Autodesk Inventor part; units mm, degrees
ref_plane "YZ Plane" through (0, 0, 0) normal (1, 0, 0) x (0, 1, 0)
ref_plane "XZ Plane" through (0, 0, 0) normal (0, 1, 0) x (-1, 0, 0)
ref_plane "XY Plane" through (0, 0, 0) normal (0, 0, 1) x (1, 0, 0)
sketch "Motor_Lego_Axle_Connector" plane through (0, 0, 0) normal (0, 0, 1) x (1, 0, 0)
  circle A0 centre (0, 0) radius 4.5
  circle A1 centre (0, 0) radius 2.7
  line L0 (-1.8, 2.0125) -> (-1.8, -2.0125)
  line L1 (0, 4.5) -> (0, -4.5) construction
  line L2 (1.8, 2.0125) -> (1.8, -2.0125)
  line L3 (0.9, 2.4) -> (-0.9, 2.4)
  line L4 (0.9, 2.4) -> (0.9, 1.4)
  line L5 (1.4, 1.4) -> (0.9, 1.4) construction
  line L6 (1.4, 1.4) -> (1.4, 0.9) construction
  arc A2 (0.9, 1.4) -> (1.4, 0.9) centre (1.4, 1.4) ccw
  line L7 (1.4, 0.9) -> (2.4, 0.9)
  line L8 (-0.9, 1.4) -> (-0.9, 2.4)
  arc A3 (-1.4, 0.9) -> (-0.9, 1.4) centre (-1.4, 1.4) ccw
  line L9 (-2.4, 0.9) -> (-1.4, 0.9)
  line L10 (-2.4, 0.9) -> (-2.4, -0.9)
  line L11 (-1.4, -0.9) -> (-2.4, -0.9)
  arc A4 (-0.9, -1.4) -> (-1.4, -0.9) centre (-1.4, -1.4) ccw
  line L12 (-0.9, -2.4) -> (-0.9, -1.4)
  line L13 (-0.9, -2.4) -> (0.9, -2.4)
  line L14 (0.9, -1.4) -> (0.9, -2.4)
  arc A5 (1.4, -0.9) -> (0.9, -1.4) centre (1.4, -1.4) ccw
  line L15 (2.4, -0.9) -> (1.4, -0.9)
  line L16 (2.4, -0.9) -> (2.4, 0.9)
  point P0 (1.8, -2.0125)
  point P1 (0, 2.4)
  point P2 (-2.4, 0)
  point P3 (0, -2.4)
  point P4 (2.4, 0)
  dimension "d0" = 9
  dimension "d1" = 5.4
  dimension "d2" = 9
  dimension "d3" = 1.8
  dimension "d12" = 1.8
  dimension "d13" = 2.4
  dimension "d14" = 1
  dimension "d16" = 0.5
  dimension "d17" = 1
  dimension "d20" = 360
extrude "Motor_Side_Outer_Ring_Extrusion" add sketch "Motor_Lego_Axle_Connector" along normal blind 9
extrude "Motor_Connector_Extrusion" add sketch "Motor_Lego_Axle_Connector" along normal blind 7.9 separate body contours A1 L2 L15 L16 L7 | L0 L9 L10 L11 A1 | L7 L16 L15 L2 | L0 L11 L10 L9
extrude "Seperation_Extrusion" add sketch "Motor_Lego_Axle_Connector" against normal blind 3 contours A1 L2 L15 L16 L7 | L2 L7 A2 L4 L3 L8 A3 L9 L0 A1 | A1 L0 L11 A4 L12 L13 L14 A5 L15 L2 | L0 L9 L10 L11 A1 | L7 L16 L15 L2 | L2 L15 A5 L14 L13 L12 A4 L11 L0 L9 A3 L8 L3 L4 A2 L7 | L0 L11 L10 L9
extrude "Lego_Axle_Side_Outer_Ring_Extrusion" add sketch "Motor_Lego_Axle_Connector" against normal blind 11
extrude "Lego_Axle_Connector_Extrusion" add sketch "Motor_Lego_Axle_Connector" against normal blind 11 contours A1 L2 L15 L16 L7 | L2 L7 A2 L4 L3 L8 A3 L9 L0 A1 | A1 L0 L11 A4 L12 L13 L14 A5 L15 L2 | L0 L9 L10 L11 A1
equation "\"d2\" = d0"
properties part number "Motor_Lego_Axle_Connector"
Source: CAD feature listing. Evaluate the final solid. Frame: model axes, mm. A direction names the side the tool comes from. Coordinates: 2 decimals unless noted, no trailing zeros. Loops run counter-clockwise (first coordinate to the right, second up) from the corner with the lowest first, then second, coordinate; pieces in that order, holes last. Notation, with made-up numbers: (43, 72) -> (92, 72) arc R29 cw to (92, 98) -> close; hole circle Ø8 at (48.5, -5). An arc over 180 degrees is marked (long way). One line per item, written item: value. Start each with the question number.
Q1. Section query C-C, the plane x = 0. Return the cut outline in (y, z), and give its area (3 significant figures).
Q2. Section query D-D, the plane z = -0.75. Return the cut outline in (x, y), and give its area (3 significant figures).
Q3. Line query: line 1 along Y through (x, z) = (0, 7); line 2 along X through (y, z) = (2.25, 6.75); line 3 along X through (y, z) = (-0.75, 5.75). Output: solid intervals per line, ascending.
Q4. Mould query, pull axis X, two halves, no side actions, for faces 4 (the face through (-0.59, 4.46, -0.86)), 5 (the face through (-0.9, 2, -7)), 6 (the face through (-1.1, -1.9, -11)). Classes: pulls with the +X half, pulls with the -X half, needs draft (parallel to the pull), parting line crosses it, or undercut.
Q5. Section query A-A, the plane z = -6.5. Return the cut outline in (x, y), and give its area (3 significant figures).
Q6. Contact query for flat-ended pins moving along their axis: P1, Ø0.8, axis at x = 2, z = -7, coming from the -Y side; P2, Ø1, axis at x = 2.5, z = -1, coming from the -Y side; P3, Ø1.1, axis at x = -0.5, y = -1, coming from the +Z side; P4, Ø2, axis at x = -1, z = 6.5, coming from the +Y side. Output: stop coordinate, or through.
Q7. Set-up query: faces 1 (the face through (0, -3, 9)), 2 (the face through (-2, 0, 7.9)), 3 (the face through (2, 0.9, -7)). Return all of +Z, -Z, +X, -X, +Y, -Y with unobstructed straight access to the full face (end or side cutting, diameter ignored); none if empty.
Q8. Section query B-B, the plane y = 0. Return the cut outline in (x, z).
Results:
1. outline: (-4.5, -11) -> (-2.4, -11) -> (-2.4, -3) -> (2.4, -3) -> (2.4, -11) -> (4.5, -11) -> (4.5, 9) -> (2.7, 9) -> (2.7, 0) -> (-2.7, 0) -> (-2.7, 9) -> (-4.5, 9) -> close
1. area: 93.0 mm^2
2. outline: circle Ø9 at (0, 0)
2. area: 63.6 mm^2
3. line 1: -4.5 to -2.7, 2.7 to 4.5
3. line 2: -3.9 to -1.49, 1.49 to 3.9
3. line 3: -4.44 to -1.8, 1.8 to 4.44
4. face 4: parting line crosses it
4. face 5: undercut
4. face 6: needs draft
5. outline: circle Ø9 at (0, 0); hole (-2.4, -0.9) -> (-1.4, -0.9) arc R0.5 cw to (-0.9, -1.4) -> (-0.9, -2.4) -> (0.9, -2.4) -> (0.9, -1.4) arc R0.5 cw to (1.4, -0.9) -> (2.4, -0.9) -> (2.4, 0.9) -> (1.4, 0.9) arc R0.5 cw to (0.9, 1.4) -> (0.9, 2.4) -> (-0.9, 2.4) -> (-0.9, 1.4) arc R0.5 cw to (-1.4, 0.9) -> (-2.4, 0.9) -> close
5. area: 49.4 mm^2
6. P1: y = -4.21
6. P2: y = -4.03
6. P3: z = 0
6. P4: y = 4.5
7. face 1: +Z, +X, -X, +Y, -Y
7. face 2: +Z
7. face 3: -Z
8. outline: (-4.5, -11) -> (-2.4, -11) -> (-2.4, -3) -> (2.4, -3) -> (2.4, -11) -> (4.5, -11) -> (4.5, 9) -> (2.7, 9) -> (2.7, 7.9) -> (1.8, 7.9) -> (1.8, 0) -> (-1.8, 0) -> (-1.8, 7.9) -> (-2.7, 7.9) -> (-2.7, 9) -> (-4.5, 9) -> close
